Autodesk Inventor part; units mm, degrees
ref_plane "YZ Plane" through (0, 0, 0) normal (1, 0, 0) x (0, 1, 0)
ref_plane "XZ Plane" through (0, 0, 0) normal (0, 1, 0) x (-1, 0, 0)
ref_plane "XY Plane" through (0, 0, 0) normal (0, 0, 1) x (1, 0, 0)
sketch "Sketch1" plane through (0, 0, 0) normal (0, 0, 1) x (1, 0, 0)
  line L0 (0, 0) -> (30, 0)
  line L1 (30, 0) -> (30, 9)
  line L2 (30, 9) -> (0, 9)
  line L3 (0, 9) -> (0, 0)
  circle A0 centre (-5.5, 5.099) radius 7.5 construction
  circle A1 centre (-5.5, 5.099) radius 4 construction
  circle A2 centre (14.5, 5.099) radius 2.75
  circle A3 centre (24.5, 4.5) radius 2.25
  circle A4 centre (4.5, 4.5) radius 2.25
  point P0 (-11, 0)
  point P1 (30, 4.5)
  dimension "d0" = 9
  dimension "d1" = 30
  dimension "d2" = 15
  dimension "d3" = 8
  dimension "d4" = 11
  dimension "d5" = 5.5
  dimension "d6" = 4.5
  dimension "d7" = 4.5
  dimension "d8" = 5.5
  dimension "d9" = 10
  dimension "d10" = 10
extrude "Extrusion1" add sketch "Sketch1" along normal blind 6.5
sketch "Sketch2" plane through (0, 0, 6.5) normal (0, 0, 1) x (1, 0, 0)
  line L0 (0, 0) -> (30, 0)
  line L1 (30, 0) -> (30, 9)
  line L2 (30, 9) -> (0, 9)
  line L3 (8, 0) -> (16, 0)
  line L4 (16, 0) -> (16, -4.5)
  line L5 (14, -6.5) -> (10, -6.5)
  line L6 (8, -4.5) -> (8, 0)
  arc A0 (8, -4.5) -> (10, -6.5) centre (10, -4.5) ccw
  arc A1 (14, -6.5) -> (16, -4.5) centre (14, -4.5) ccw
  line L7 (10.5, 9) -> (18.5, 9)
  line L8 (18.5, 9) -> (18.5, 15)
  line L9 (16.5, 17) -> (12.5, 17)
  line L10 (10.5, 15) -> (10.5, 9)
  arc A2 (12.5, 17) -> (10.5, 15) centre (12.5, 15) ccw
  arc A3 (18.5, 15) -> (16.5, 17) centre (16.5, 15) ccw
  dimension "d13" = 2
  dimension "d14" = 8
  dimension "d15" = 6.5
  dimension "d16" = 14
  dimension "d17" = 2
  dimension "d18" = 8
  dimension "d19" = 8
  dimension "d20" = 11.5
extrude "Extrusion2" add sketch "Sketch2" against normal blind 6.5
properties part number "x_motor_lower_nut_stop" material "Plywood, Finish"
The model under review builds one solid part; all positions refer to its coordinate system, in mm. A direction names the side the tool comes from. Coordinates: 2 decimals unless noted, no trailing zeros. Write each loop counter-clockwise with the first axis right and the second up, starting at its lowest first coordinate (ties: lowest second). Pieces come first, ordered by that corner, then holes. Notation, with made-up numbers: (79.25, -24) -> (129.25, -24) arc R9 cw to (129.25, -8) -> close; hole circle Ø1 at (21, -20.5). An arc over 180 degrees is marked (long way). One line per item, written item: value. Start each with the question number.
Q1. To check wall thickness, follow probe 1 along Y at (x, z) = (4.5, 3.5); probe 2 along X at (y, z) = (5.5, 4); probe 3 along X at (y, z) = (12.75, 3.25). State the ranges of each line that lie inside material, in increasing order.
Q2. Add section C-C, the plane z = 5. Give the boundary of the cut face in (x, y).
Q3. For faces 5 (the face through (23, 0, 3)), 6 (the face through (24, 9, 3)), 7 (the face through (8.57, -5.9, 3.3)), list the 3-axis set-ups (+Z, -Z, +X, -X, +Y, -Y) from which the entire face can be reached by the end or side of a thin tool; tool diameter is ignored.
Q4. Add section B-B, the plane y = 4.5. Give the boundary of the cut face in (x, z), then the cut area to 3 significant figures.
Q5. Add section A-A, the plane x = 24.5. Give the boundary of the cut face in (y, z).
Q6. Clearance check with flat-ended pins moving along their axes: P1, Ø1, axis at y = 13, z = 5.5, coming from the +X side; P2, Ø3.5, axis at y = -2.5, z = 3, coming from the +X side; P3, Ø6, axis at x = 4.5, y = 4.5, coming from the +Z side; P4, Ø1.3, axis at y = -1.5, z = 5, coming from the -X side. State where each tip first meets the part, or that it passes through.
Q7. Add section D-D, the plane x = 19.75. Give the boundary of the cut face in (y, z).
Q8. The part is to be moulded in two halves that separate along Y. For faces 1 (the face through (10.5, 12, 3)), 2 (the face through (11.753, 4.978, 3.204)), 3 (the face through (26.646, 3.824, 3.204)), 4 (the face through (4, 0, 3)), say which applies: +Y half, -Y half, draft (parallel to the pull), parting line (faces both ways), or undercut.
Response:
1. probe 1: 0 to 2.25, 6.75 to 9
1. probe 2: 0 to 2.48, 6.52 to 11.78, 17.22 to 22.48, 26.52 to 30
1. probe 3: 10.5 to 18.5
2. outline: (0, 0) -> (8, 0) -> (8, -4.5) arc R2 ccw to (10, -6.5) -> (14, -6.5) arc R2 ccw to (16, -4.5) -> (16, 0) -> (30, 0) -> (30, 9) -> (18.5, 9) -> (18.5, 15) arc R2 ccw to (16.5, 17) -> (12.5, 17) arc R2 ccw to (10.5, 15) -> (10.5, 9) -> (0, 9) -> close; hole circle Ø4.5 at (4.5, 4.5); hole circle Ø5.5 at (14.5, 5.1); hole circle Ø4.5 at (24.5, 4.5)
3. face 5: +Z, -Z, +X, -Y
3. face 6: +Z, -Z, +X, +Y
3. face 7: +Z, -Z, -X, -Y
4. outline: (0, 0) -> (2.25, 0) -> (2.25, 6.5) -> (0, 6.5) -> close; (6.75, 0) -> (11.82, 0) -> (11.82, 6.5) -> (6.75, 6.5) -> close; (17.18, 0) -> (22.25, 0) -> (22.25, 6.5) -> (17.18, 6.5) -> close; (26.75, 0) -> (30, 0) -> (30, 6.5) -> (26.75, 6.5) -> close
4. area: 102 mm²
5. outline: (0, 0) -> (2.25, 0) -> (2.25, 6.5) -> (0, 6.5) -> close; (6.75, 0) -> (9, 0) -> (9, 6.5) -> (6.75, 6.5) -> close
6. P1: x = 18.5
6. P2: x = 16
6. P3: z = 6.5
6. P4: x = 8
7. outline: (0, 0) -> (9, 0) -> (9, 6.5) -> (0, 6.5) -> close
8. face 1: draft
8. face 2: undercut
8. face 3: undercut
8. face 4: -Y half
